Drawing for the job (mm, zero at the part's lowest x, y, z). A direction names the side the tool comes from. Give positions to 0.01 mm unless a question says otherwise; leave off trailing zeros. Order: outer loops, then holes, each group sorted by start corner. A loop starts at its lowest first (then second) coordinate and runs counter-clockwise, first axis right, second up. Notation, with made-up numbers: (-8.75, 36) - (30.25, 36) arc R26 ccw to (30.25, 70) - close; hole circle Ø5 at (10.5, 63). An arc over 180 degrees is marked (long way). Use a Markdown table: item, result.
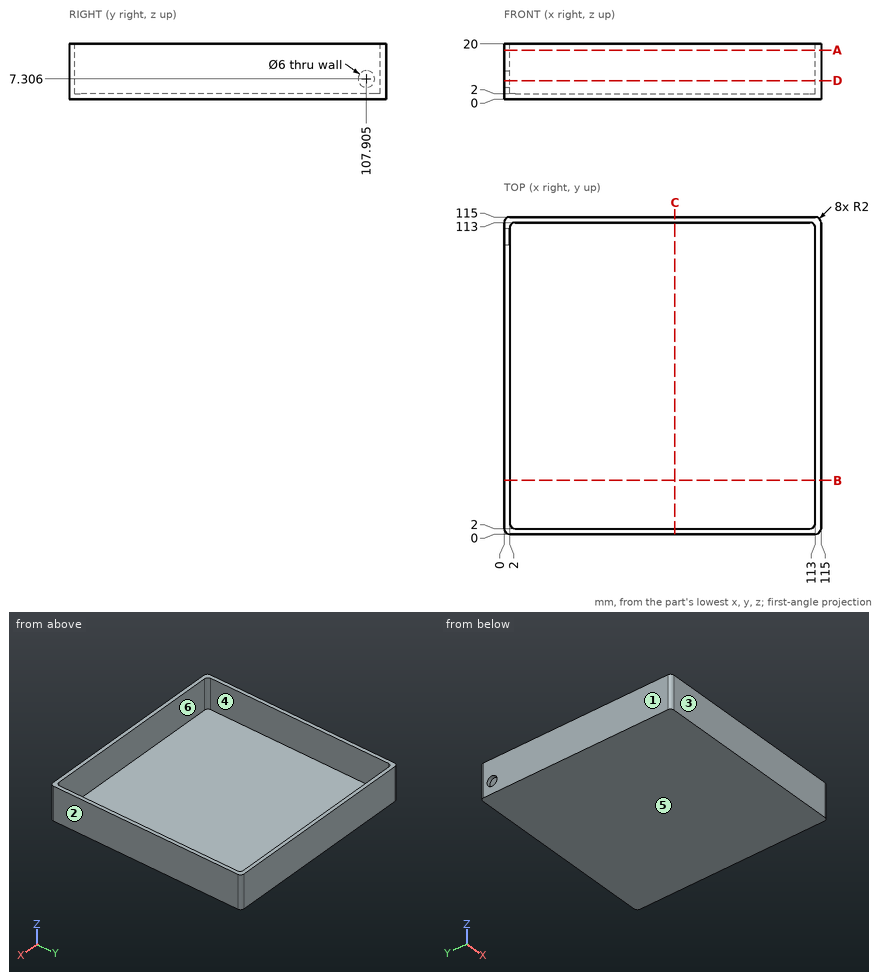
1) Slice it at D-D (z = 6.75). Write the cut outline in (x, y).
Computed:
| item | result |
|---|---|
| outline | (0, 2) arc R2 ccw to (2, 0) - (113, 0) arc R2 ccw to (115, 2) - (115, 113) arc R2 ccw to (113, 115) - (2, 115) arc R2 ccw to (0, 113) - (0, 110.85) - (2, 110.85) - (2, 111) arc R2 cw to (4, 113) - (111, 113) arc R2 cw to (113, 111) - (113, 4) arc R2 cw to (111, 2) - (4, 2) arc R2 cw to (2, 4) - (2, 104.96) - (0, 104.96) - close |
2) Slice it at B-B (y = 19.5). Write the cut outline in (x, z), and give its area (3 significant figures).
Computed:
| item | result |
|---|---|
| outline | (0, 0) - (115, 0) - (115, 20) - (113, 20) - (113, 2) - (2, 2) - (2, 20) - (0, 20) - close |
| area | 302 mm² |
3) Pin check, flat tip, straight feed: P1, Ø3, axis at x = 42, y = 44.5, coming from the +Z side. Stop position of the tip, or through.
Computed:
| item | result |
|---|---|
| P1 | stops at z = 2 |
4) Tool access for the marked faces 5 and 6: list every direction of +Z, -Z, +X, -X, +Y, -Y with a clear straight run to the whole face (end or side of a thin tool).
Computed:
| item | result |
|---|---|
| face 5 | -Z, +X, -X, +Y, -Y |
| face 6 | +Z |
5) Slice it at A-A (z = 17.75). Write the cut outline in (x, y).
Computed:
| item | result |
|---|---|
| outline | (0, 2) arc R2 ccw to (2, 0) - (113, 0) arc R2 ccw to (115, 2) - (115, 113) arc R2 ccw to (113, 115) - (2, 115) arc R2 ccw to (0, 113) - close; hole (2, 4) arc R2 ccw to (4, 2) - (111, 2) arc R2 ccw to (113, 4) - (113, 111) arc R2 ccw to (111, 113) - (4, 113) arc R2 ccw to (2, 111) - close |
6) Wall check: line 1 (Y direction, x = 69, z = 15.25); line 2 (Z direction, x = 104, y = 97). Give the ranges that are in metal, low to high. Write a range as from..to.
Computed:
| item | result |
|---|---|
| line 1 | y = 0..2, 113..115 |
| line 2 | z = 0..2 |
7) Two-plate mould, pull along X, no slides. Class the marked faces 1, 2, 3 and 4: +X half, -X half, draft (parallel to the pull), parting line (faces both ways), or undercut.
Computed:
| item | result |
|---|---|
| face 1 | -X half |
| face 2 | +X half |
| face 3 | draft |
| face 4 | undercut |
